```python
from build123d import *

# Parameters (mm, degrees)
F0_W         = 243
F0_H         = 177
F1_DEPTH     = 8.1
F2_R         = 14
F3_W         = 16.2
F3_H         = 5.2
F4_DEPTH     = 0.2
F5_R         = 2
F6_R         = 4
F7_T1_DEPTH  = 12.2
F7_T3_DEPTH  = 1.2
F7_T6_ANGLE  = 90
F7_T8_ANGLE  = 90
F7_T10_ANGLE = 90
F7_T12_ANGLE = 90
F7_T13_DEPTH = 215
F7_T15_DEPTH = 149
F7_T18_ANGLE = 90
F7_T20_ANGLE = 90
F7_T22_ANGLE = 90
F7_T24_ANGLE = 90


# Not quite as in the source:
# - a fillet or chamfer that OpenCascade refuses, or shapes differently, is made with other operations: its cross-section is extruded or revolved along the edge and cut away or added


with BuildPart() as f1:
    # F0 (on Top) → F1 (new body)
    with BuildSketch(Plane.XY):
        with Locations((0, 88.5)):
            Rectangle(F0_W, F0_H)
    extrude(amount=F1_DEPTH)

    # F2
    f2_edges = [f1.edges().sort_by_distance(p)[0] for p in [
        (-121.5, 0, 4.05),
        (121.5, 0, 4.05),
        (121.5, 177, 4.05),
        (-121.5, 177, 4.05),
    ]]
    fillet(f2_edges, radius=F2_R)

    # F3 (on face) → F4 (join)
    with BuildSketch(Plane.XY.offset(8.1)):
        with Locations((0, 8.6)):
            Rectangle(F3_W, F3_H)
    extrude(amount=F4_DEPTH)

    # F5
    f5_edges = [f1.edges().sort_by_distance(p)[0] for p in [
        (8.1, 6, 8.2),
        (8.1, 11.2, 8.2),
        (-8.1, 6, 8.2),
        (-8.1, 11.2, 8.2),
    ]]
    fillet(f5_edges, radius=F5_R)

    # F6
    f6_edges = [f1.edges().sort_by_distance(p)[0] for p in [
        (121.5, 88.5, 0),
        (0, 177, 0),
        (117.399495, 172.899495, 0),
        (-117.399495, 172.899495, 0),
        (-121.5, 88.5, 0),
        (117.399495, 4.100505, 0),
        (-117.399495, 4.100505, 0),
        (0, 0, 0),
    ]]
    fillet(f6_edges, radius=F6_R)

    # F7: fillet of radius 1 on 16 edges, made by hand

    # F7_s2 → F7_t1 (join)
    with BuildSketch(Plane.YZ.offset(-6.1)):
        with BuildLine():
            ThreePointArc((11.8, 8.1), (11.483772234, 8.1513167019), (11.2, 8.3))
            Line((11.2, 8.3), (11.2, 8.1))
            Line((11.2, 8.1), (11.8, 8.1))
        make_face()
        with BuildLine():
            ThreePointArc((5.4, 8.1), (5.716227766, 8.1513167019), (6, 8.3))
            Line((6, 8.3), (6, 8.1))
            Line((6, 8.1), (5.4, 8.1))
        make_face()
    extrude(amount=F7_T1_DEPTH)

    # F7_s4 → F7_t3 (join)
    with BuildSketch(Plane.XZ.offset(-9.2)):
        with BuildLine():
            ThreePointArc((8.7, 8.1), (8.383772234, 8.1513167019), (8.1, 8.3))
            Line((8.1, 8.3), (8.1, 8.1))
            Line((8.1, 8.1), (8.7, 8.1))
        make_face()
        with BuildLine():
            ThreePointArc((-8.7, 8.1), (-8.383772234, 8.1513167019), (-8.1, 8.3))
            Line((-8.1, 8.3), (-8.1, 8.1))
            Line((-8.1, 8.1), (-8.7, 8.1))
        make_face()
    extrude(amount=F7_T3_DEPTH)

    # F7_s5 → F7_t6 (revolve)
    with BuildSketch(Plane.YZ.offset(6.1)):
        with BuildLine():
            ThreePointArc((11.8, 8.1), (11.483772234, 8.1513167019), (11.2, 8.3))
            Line((11.2, 8.3), (11.2, 8.1))
            Line((11.2, 8.1), (11.8, 8.1))
        make_face()
    revolve(axis=Axis((6.1, 9.2, 8.1), (0, 0, -1)), revolution_arc=F7_T6_ANGLE)

    # F7_s7 → F7_t8 (revolve)
    with BuildSketch(Plane.YZ.offset(-6.1)):
        with BuildLine():
            ThreePointArc((11.8, 8.1), (11.483772234, 8.1513167019), (11.2, 8.3))
            Line((11.2, 8.3), (11.2, 8.1))
            Line((11.2, 8.1), (11.8, 8.1))
        make_face()
    revolve(axis=Axis((-6.1, 9.2, 8.1), (0, 0, 1)), revolution_arc=F7_T8_ANGLE)

    # F7_s9 → F7_t10 (revolve)
    with BuildSketch(Plane.YZ.offset(6.1)):
        with BuildLine():
            ThreePointArc((5.4, 8.1), (5.716227766, 8.1513167019), (6, 8.3))
            Line((6, 8.3), (6, 8.1))
            Line((6, 8.1), (5.4, 8.1))
        make_face()
    revolve(axis=Axis((6.1, 8, 8.1), (0, 0, 1)), revolution_arc=F7_T10_ANGLE)

    # F7_s11 → F7_t12 (revolve)
    with BuildSketch(Plane.XZ.offset(-8)):
        with BuildLine():
            ThreePointArc((-8.7, 8.1), (-8.383772234, 8.1513167019), (-8.1, 8.3))
            Line((-8.1, 8.3), (-8.1, 8.1))
            Line((-8.1, 8.1), (-8.7, 8.1))
        make_face()
    revolve(axis=Axis((-6.1, 8, 8.1), (0, 0, 1)), revolution_arc=F7_T12_ANGLE)

    # F7_s14 → F7_t13 (cut)
    with BuildSketch(Plane.YZ.offset(-107.5)):
        with BuildLine():
            ThreePointArc((177, 7.1), (176.7071067812, 7.8071067812), (176, 8.1))
            Line((176, 8.1), (177, 8.1))
            Line((177, 8.1), (177, 7.1))
        make_face()
        with BuildLine():
            ThreePointArc((1, 8.1), (0.2928932188, 7.8071067812), (0, 7.1))
            Line((0, 7.1), (0, 8.1))
            Line((0, 8.1), (1, 8.1))
        make_face()
    extrude(amount=F7_T13_DEPTH, mode=Mode.SUBTRACT)

    # F7_s16 → F7_t15 (cut)
    with BuildSketch(Plane.XZ.offset(-163)):
        with BuildLine():
            ThreePointArc((120.5, 8.1), (121.2071067812, 7.8071067812), (121.5, 7.1))
            Line((121.5, 7.1), (121.5, 8.1))
            Line((121.5, 8.1), (120.5, 8.1))
        make_face()
        with BuildLine():
            ThreePointArc((-120.5, 8.1), (-121.2071067812, 7.8071067812), (-121.5, 7.1))
            Line((-121.5, 7.1), (-121.5, 8.1))
            Line((-121.5, 8.1), (-120.5, 8.1))
        make_face()
    extrude(amount=F7_T15_DEPTH, mode=Mode.SUBTRACT)

    # F7_s17 → F7_t18 (revolve, cut)
    with BuildSketch(Plane.YZ.offset(107.5)):
        with BuildLine():
            ThreePointArc((177, 7.1), (176.7071067812, 7.8071067812), (176, 8.1))
            Line((176, 8.1), (177, 8.1))
            Line((177, 8.1), (177, 7.1))
        make_face()
    revolve(axis=Axis((107.5, 163, 8.1), (0, 0, -1)), revolution_arc=F7_T18_ANGLE, mode=Mode.SUBTRACT)

    # F7_s19 → F7_t20 (revolve, cut)
    with BuildSketch(Plane.YZ.offset(-107.5)):
        with BuildLine():
            ThreePointArc((176, 8.1), (176.7071067812, 7.8071067812), (177, 7.1))
            Line((177, 7.1), (177, 8.1))
            Line((177, 8.1), (176, 8.1))
        make_face()
    revolve(axis=Axis((-107.5, 163, 8.1), (0, 0, 1)), revolution_arc=F7_T20_ANGLE, mode=Mode.SUBTRACT)

    # F7_s21 → F7_t22 (revolve, cut)
    with BuildSketch(Plane.YZ.offset(107.5)):
        with BuildLine():
            ThreePointArc((1, 8.1), (0.2928932188, 7.8071067812), (0, 7.1))
            Line((0, 7.1), (0, 8.1))
            Line((0, 8.1), (1, 8.1))
        make_face()
    revolve(axis=Axis((107.5, 14, 8.1), (0, 0, 1)), revolution_arc=F7_T22_ANGLE, mode=Mode.SUBTRACT)

    # F7_s23 → F7_t24 (revolve, cut)
    with BuildSketch(Plane.XZ.offset(-14)):
        with BuildLine():
            ThreePointArc((-120.5, 8.1), (-121.2071067812, 7.8071067812), (-121.5, 7.1))
            Line((-121.5, 7.1), (-121.5, 8.1))
            Line((-121.5, 8.1), (-120.5, 8.1))
        make_face()
    revolve(axis=Axis((-107.5, 14, 8.1), (0, 0, 1)), revolution_arc=F7_T24_ANGLE, mode=Mode.SUBTRACT)


solid = f1.part
```
Input: part model. Units: mm. Frame: model coordinates. Coordinates: 2 decimals unless noted, no trailing zeros. Loops run counter-clockwise (first coordinate to the right, second up) from the corner with the lowest first, then second, coordinate; pieces in that order, holes last. Notation, with made-up numbers: (70, 70) -> (111, 70) arc R25 ccw to (111, 84) -> close; hole circle Ø1 at (15.25, 27). An arc over 180 degrees is marked (long way). Use a Markdown table: item, result.
1) Cut plane A-A (y = 31). Return the cut outline in (x, z), then the cut area to 3 significant figures.
Results found:
| item | result |
|---|---|
| outline | (-121.5, 4) arc R4 ccw to (-117.5, 0) -> (117.5, 0) arc R4 ccw to (121.5, 4) -> (121.5, 7.1) arc R1 ccw to (120.5, 8.1) -> (-120.5, 8.1) arc R1 ccw to (-121.5, 7.1) -> close |
| area | 1,960 mm2 |
2) Material intervals for line 1 along Z through (x, y) = (-101.5, 35); line 2 along Y through (x, z) = (108, 5.5); line 3 along X through (y, z) = (131, 7.5), sorted ascending. Write a range as from..to.
Results found:
| item | result |
|---|---|
| line 1 | z = 0..8.1 |
| line 2 | y = 0.01..176.99 |
| line 3 | x = -121.42..121.42 |
3) Contact query for a flat-ended pin moving along its axis: pin 1 (8 mm diameter, centred on x = 14.5, y = 61, fed in from +Z). Output: stop coordinate, or through.
Results found:
| item | result |
|---|---|
| pin 1 | stops at z = 8.1 |
4) Cut plane B-B (x = 49.5). Return the cut outline in (y, z).
Results found:
| item | result |
|---|---|
| outline | (0, 4) arc R4 ccw to (4, 0) -> (173, 0) arc R4 ccw to (177, 4) -> (177, 7.1) arc R1 ccw to (176, 8.1) -> (1, 8.1) arc R1 ccw to (0, 7.1) -> close |
